from build123d import *

# Parameters (mm, degrees)
F0_W     = 300
F0_H     = 150
F1_DEPTH = 35
F2_R     = 30
F3_R     = 9.6568542495
F4_T     = -2.5
F5_R     = 46.3829958517
F6_DEPTH = 14


with BuildPart() as f1:
    # F0 (on Top) → F1 (new body, symmetric)
    with BuildSketch(Plane.XY):
        with Locations((1.3466058194, -4.4853053987)):
            Rectangle(F0_W, F0_H)
    extrude(amount=F1_DEPTH, both=True)

    # F2
    f2_edges = [f1.edges().sort_by_distance(p)[0] for p in [
        (-148.653394, 70.514695, 0),
    ]]
    fillet(f2_edges, radius=F2_R)

    # F3
    f3_edges = [f1.edges().sort_by_distance(p)[0] for p in [
        (16.346606, 70.514695, 35),
    ]]
    fillet(f3_edges, radius=F3_R)

    # F4
    f4_openings = [f1.faces().sort_by_distance(p)[0] for p in [
        (1.487632, -79.485305, -0.031329),
    ]]
    offset(amount=F4_T, openings=f4_openings)

    # F5 (on face) → F6 (cut)
    with BuildSketch(Plane(origin=(0, 0, -35), x_dir=(1, 0, 0), z_dir=(0, 0, -1))):
        with Locations((-76.8001675606, 0)):
            Circle(F5_R)
    extrude(amount=-F6_DEPTH, mode=Mode.SUBTRACT)


solid = f1.part
Source: CAD feature listing. Evaluate the final solid. Frame: model axes, mm. A direction names the side the tool comes from. Give positions to 0.01 mm unless a question says otherwise; leave off trailing zeros. Write each loop counter-clockwise with the first axis right and the second up, starting at its lowest first coordinate (ties: lowest second). Pieces come first, ordered by that corner, then holes. Notation, with made-up numbers: M 87.25,55.25 L 125.25,55.25 A30 cw 125.25,91.25 Z; hole C -15.5,-10.75 d2. An arc over 180 degrees is marked long. Return JSON: item names as keys, results as strings. Group by question number.
1) Cut plane D-D, the plane x = -71. Output: boundary loops of the cut face in (y, z).
2) Draft query along Z for faces 1 (the face through (4, -8, 35)), 2 (the face through (151.347, -6, 0)), 3 (the face through (-1, -5, -32.5)), 4 (the face through (16.97, 65.86, 30.46)). Return one class per face: released by +Z, released by -Z, zero draft, split by the parting line, or undercut.
3) Cut plane B-B, the plane x = 44. Output: boundary loops of the cut face in (y, z).
4) Cut plane C-C, the plane z = 8.5. Output: boundary loops of the cut face in (x, y), then the cut area to 3 significant figures.
5) Cut plane A-A, the plane y = -65.5. Output: boundary loops of the cut face in (x, z), then the cut area to 3 significant figures.
6) Ray query, L1, parallel to X at y = -57, z = -11.5; L2, parallel to Z at x = 126.5, y = -32.5; L3, parallel to X at y = 0, z = -34.1. Return the intervals inside material, ascending.
7) Set-up query: faces 5 (the face through (13, 68.015, -3)), 6 (the face through (1, -79.485, -34)), 7 (the face through (-33.95, 17.76, -33.77)). Return all of +Z, -Z, +X, -X, +Y, -Y with unobstructed straight access to the full face (end or side cutting, diameter ignored); none if empty.
8) First-contact query: pin 1 Ø3 at (x, z) = (-34.5, 25.5) entering from -Y; pin 2 Ø12 at (x, z) = (-85, 22) entering from -Y; pin 3 Ø1.5 at (x, z) = (79.5, -11) entering from -Y. Flat tips, straight axial feed; report the tip coordinate or a pass-through.
Data:
{
 "1": {"outline": "M -79.49,-35 L -46.02,-35 L -46.02,-32.5 L -79.49,-32.5 Z; M -79.49,32.5 L 60.86,32.5 A7.16 cw 68.01,25.34 L 68.01,-32.5 L 46.02,-32.5 L 46.02,-35 L 70.51,-35 L 70.51,25.34 A9.66 ccw 60.86,35 L -79.49,35 Z"},
 "2": {"face 1": "released by +Z", "face 2": "zero draft", "face 3": "undercut", "face 4": "undercut"},
 "3": {"outline": "M -79.49,-35 L 70.51,-35 L 70.51,25.34 A9.66 ccw 60.86,35 L -79.49,35 L -79.49,32.5 L 60.86,32.5 A7.16 cw 68.01,25.34 L 68.01,-32.5 L -79.49,-32.5 Z"},
 "4": {"outline": "M -148.65,-79.49 L -146.15,-79.49 L -146.15,40.51 A27.5 cw -118.65,68.01 L 148.85,68.01 L 148.85,-79.49 L 151.35,-79.49 L 151.35,70.51 L -118.65,70.51 A30 ccw -148.65,40.51 Z", "area": "1,460 mm²"},
 "5": {"outline": "M -148.65,-35 L 151.35,-35 L 151.35,35 L -139,35 A9.66 ccw -148.65,25.34 Z; hole M -146.15,-32.5 L 148.85,-32.5 L 148.85,32.5 L -139,32.5 A7.16 ccw -146.15,25.34 Z", "area": "1,820 mm²"},
 "6": {"L1": "x = -148.65 to -146.15, 148.85 to 151.35", "L2": "z = -35 to -32.5, 32.5 to 35", "L3": "x = -148.65 to -123.18, -30.42 to 151.35"},
 "7": {"face 5": "-Y", "face 6": "+Z, -Z, +X, -X, -Y", "face 7": "-Z"},
 "8": {"pin 1": "stops at y = 67.82", "pin 2": "stops at y = 67.5", "pin 3": "stops at y = 68.01"}
}
